Verification items for the finished model (mm, model axes). Face numbers are marked on the shaded views. A direction names the side the tool comes from. Coordinates: 2 decimals unless noted, no trailing zeros. Write each loop counter-clockwise with the first axis right and the second up, starting at its lowest first coordinate (ties: lowest second). Pieces come first, ordered by that corner, then holes. Notation, with made-up numbers: (8.25, 35) -> (17.25, 35) arc R18 cw to (17.25, 49) -> close; hole circle Ø1 at (9, 22.5). An arc over 180 degrees is marked (long way). Answer in a Markdown table with one row per item.
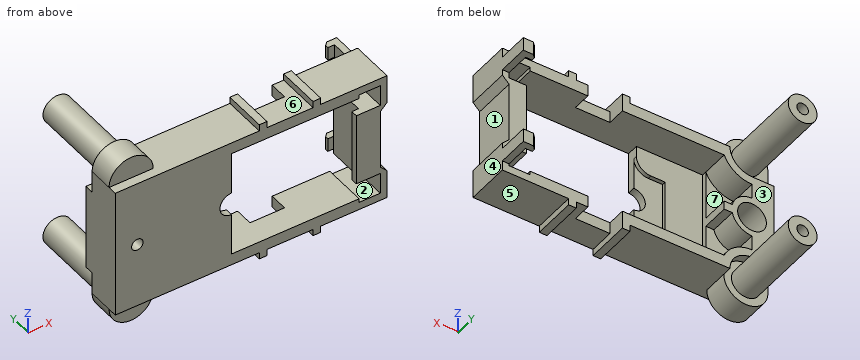
```python
from build123d import *

# Parameters (mm, degrees)
SKETCH1_W           = 35.941
SKETCH1_H           = 17.272
BOSS_EXTRUDE1_DEPTH = 5.715
SKETCH2_W           = 4.572
SKETCH2_H           = 2.413
CUT_EXTRUDE1_DEPTH  = 26.571900188
SKETCH3_W           = 4.699
SKETCH3_H           = 7.112
CUT_EXTRUDE2_DEPTH  = 21.740795338
SKETCH4_W           = 8.763
SKETCH4_H           = 14.224
CUT_EXTRUDE3_DEPTH  = 2.54
SKETCH4_2_W         = 8.763
SKETCH4_2_H         = 14.224
CUT_EXTRUDE4_DEPTH  = 4.191
SKETCH6_W           = 9.652
SKETCH6_H           = 0.8763
BOSS_EXTRUDE2_DEPTH = 0.8763
SKETCH7_W           = 0.889
SKETCH7_H           = 1.778
BOSS_EXTRUDE3_DEPTH = 4.064
SKETCH9_W           = 1.778
SKETCH9_H           = 0.8763
BOSS_EXTRUDE5_DEPTH = 0.8763
CHAMFER1_SIZE       = 0.43815
SKETCH11_W          = 1.016
SKETCH11_H          = 5.715
BOSS_EXTRUDE6_DEPTH = 0.8763
CUT_EXTRUDE5_DEPTH  = 0.508
CUT_EXTRUDE6_DEPTH  = 23.140751806
SKETCH20_W          = 5.842
SKETCH20_H          = 3.302
BOSS_EXTRUDE8_DEPTH = 4.318
CUT_EXTRUDE12_DEPTH = 1.2065
CUT_EXTRUDE13_DEPTH = 23.771103542
SKETCH26_R          = 1.905
SKETCH26_R_2        = 0.762
BOSS_EXTRUDE9_DEPTH = 11.049
SKETCH27_R          = 1.905
CUT_EXTRUDE14_DEPTH = 3.5687
SKETCH29_R          = 0.762
CUT_EXTRUDE15_DEPTH = 26.226244364


with BuildPart() as part:
    # Sketch1 → Boss-Extrude1 (new body)
    with BuildSketch(Plane(origin=(0, 0, 0), x_dir=(1, 0, 0), z_dir=(0, 1, 0))):
        Rectangle(SKETCH1_W, SKETCH1_H)
    extrude(amount=BOSS_EXTRUDE1_DEPTH)

    # Sketch2 → Cut-Extrude1 (cut, through all)
    with BuildSketch(Plane.XY.offset(8.636)):
        with Locations((4.3815, 4.5085)):
            Rectangle(SKETCH2_W, SKETCH2_H)
    extrude(amount=-CUT_EXTRUDE1_DEPTH, mode=Mode.SUBTRACT)

    # Sketch3 → Cut-Extrude2 (cut, through all)
    with BuildSketch(Plane(origin=(0, 5.715, 0), x_dir=(1, 0, 0), z_dir=(0, 1, 0))):
        with Locations((-0.254, 3.556)):
            Rectangle(SKETCH3_W, SKETCH3_H)
        Polygon((17.0815, 4.826), (17.0815, 7.62), (14.2875, 7.62), (14.2875, 7.112), (2.0955, 7.112), (2.0955, 0), (14.7955, 0), (14.7955, 4.826), align=None)
        Polygon((14.7955, -4.826), (14.7955, 0), (2.0955, 0), (2.0955, -7.112), (14.2875, -7.112), (14.2875, -7.62), (17.0815, -7.62), (17.0815, -4.826), align=None)
        with Locations((-0.254, -3.556)):
            Rectangle(SKETCH3_W, SKETCH3_H)
        Polygon((17.9705, 0), (17.0815, 0), (17.0815, -3.937), (17.9705, -4.826), align=None)
        Polygon((17.0815, 3.937), (17.0815, 0), (17.9705, 0), (17.9705, 4.826), align=None)
    extrude(amount=-CUT_EXTRUDE2_DEPTH, mode=Mode.SUBTRACT)

    # Sketch4 → Cut-Extrude3 (cut)
    with BuildSketch(Plane(origin=(0, 5.715, 0), x_dir=(1, 0, 0), z_dir=(0, 1, 0))):
        with Locations((-6.985, 0)):
            Rectangle(SKETCH4_W, SKETCH4_H)
    extrude(amount=-CUT_EXTRUDE3_DEPTH, mode=Mode.SUBTRACT)

    # Sketch4_2 → Cut-Extrude4 (cut)
    with BuildSketch(Plane(origin=(0, 5.715, 0), x_dir=(1, 0, 0), z_dir=(0, 1, 0))):
        with Locations((-6.985, 0)):
            Rectangle(SKETCH4_2_W, SKETCH4_2_H)
    extrude(amount=-CUT_EXTRUDE4_DEPTH, mode=Mode.SUBTRACT)

    # Sketch6 → Boss-Extrude2 (add)
    with BuildSketch(Plane.ZY.offset(-14.7955)):
        with Locations((0, 0.43815)):
            Rectangle(SKETCH6_W, SKETCH6_H)
    extrude(amount=BOSS_EXTRUDE2_DEPTH)

    # Sketch7 → Boss-Extrude3 (add)
    with BuildSketch(Plane(origin=(0, 5.715, 0), x_dir=(1, 0, 0), z_dir=(0, 1, 0))):
        with Locations((17.526, 6.470028065)):
            Rectangle(SKETCH7_W, SKETCH7_H)
        with Locations((17.526, -6.470028065)):
            Rectangle(SKETCH7_W, SKETCH7_H)
    extrude(amount=BOSS_EXTRUDE3_DEPTH)

    # Sketch9 → Boss-Extrude5 (add)
    with BuildSketch(Plane.ZY.offset(-17.0815)):
        with Locations((-6.470028065, 9.34085)):
            Rectangle(SKETCH9_W, SKETCH9_H)
        with Locations((6.470028065, 9.34085)):
            Rectangle(SKETCH9_W, SKETCH9_H)
    extrude(amount=BOSS_EXTRUDE5_DEPTH)

    # Chamfer1
    chamfer1_edges = [part.edges().sort_by_distance(p)[0] for p in [
        (16.2052, 9.779, -6.470028065),
        (16.2052, 9.779, 6.470028065),
    ]]
    chamfer(chamfer1_edges, length=CHAMFER1_SIZE)

    # Sketch11 → Boss-Extrude6 (add)
    with BuildSketch(Plane(origin=(0, 0, -8.636), x_dir=(-1, 0, 0), z_dir=(0, 0, -1))):
        with Locations((-1.5875, 2.8575)):
            Rectangle(SKETCH11_W, SKETCH11_H)
        with Locations((-8.6995, 2.8575)):
            Rectangle(SKETCH11_W, SKETCH11_H)
    boss_extrude6 = extrude(amount=BOSS_EXTRUDE6_DEPTH)

    # Mirror1: Boss-Extrude6 across plane
    add(boss_extrude6.mirror(Plane.XY))

    # Sketch12 → Cut-Extrude5 (cut)
    with BuildSketch(Plane(origin=(0, 1.524, 0), x_dir=(1, 0, 0), z_dir=(0, 1, 0))):
        with BuildLine():
            Line((-2.6035, -5.715), (-2.6035, 0))
            Line((-2.6035, 0), (-6.4135, 0))
            Line((-6.4135, 0), (-6.4135, -3.81))
            Line((-6.4135, -3.81), (-4.5085, -3.81))
            ThreePointArc((-4.5085, -3.81), (-3.161461582, -4.367961582), (-2.6035, -5.715))
        make_face()
        with BuildLine():
            Line((-6.4135, 0), (-2.6035, 0))
            Line((-2.6035, 0), (-2.6035, 5.715))
            ThreePointArc((-2.6035, 5.715), (-3.161461582, 4.367961582), (-4.5085, 3.81))
            Line((-4.5085, 3.81), (-6.4135, 3.81))
            Line((-6.4135, 3.81), (-6.4135, 0))
        make_face()
    extrude(amount=-CUT_EXTRUDE5_DEPTH, mode=Mode.SUBTRACT)

    # Sketch13 → Cut-Extrude6 (cut, through all)
    with BuildSketch(Plane(origin=(0, 1.016, 0), x_dir=(1, 0, 0), z_dir=(0, 1, 0))):
        with BuildLine():
            Line((-2.6035, -1.524), (-2.6035, 1.524))
            ThreePointArc((-2.6035, 1.524), (-4.1275, 0), (-2.6035, -1.524))
        make_face()
    extrude(amount=-CUT_EXTRUDE6_DEPTH, mode=Mode.SUBTRACT)

    # Sketch20 → Boss-Extrude8 (add)
    with BuildSketch(Plane.XY.offset(8.636)):
        with Locations((-15.0495, 2.8575)):
            Rectangle(SKETCH20_W, SKETCH20_H)
    boss_extrude8 = extrude(amount=BOSS_EXTRUDE8_DEPTH)

    # Mirror5: Boss-Extrude8 across plane
    add(boss_extrude8.mirror(Plane.XY))

    # Sketch23 → Cut-Extrude12 (cut)
    with BuildSketch(Plane(origin=(0, 5.715, 0), x_dir=(1, 0, 0), z_dir=(0, 1, 0))):
        with BuildLine():
            Line((-15.0495, -5.715), (-17.9705, -5.715))
            Line((-17.9705, -5.715), (-17.9705, -8.636))
            Line((-17.9705, -8.636), (-12.1285, -8.636))
            ThreePointArc((-12.1285, -8.636), (-12.984041092, -6.570541092), (-15.0495, -5.715))
        make_face()
    cut_extrude12 = extrude(amount=-CUT_EXTRUDE12_DEPTH, mode=Mode.SUBTRACT)

    # Mirror8: Cut-Extrude12 across plane
    add(cut_extrude12.mirror(Plane.XY), mode=Mode.SUBTRACT)

    # Sketch25 → Cut-Extrude13 (cut, through all)
    with BuildSketch(Plane(origin=(0, 4.5085, 0), x_dir=(1, 0, 0), z_dir=(0, 1, 0))):
        with BuildLine():
            Line((-12.1285, -8.636), (-12.1285, -12.954))
            Line((-12.1285, -12.954), (-17.9705, -12.954))
            Line((-17.9705, -12.954), (-17.9705, -8.636))
            ThreePointArc((-17.9705, -8.636), (-15.0495, -11.557), (-12.1285, -8.636))
        make_face()
    cut_extrude13 = extrude(amount=-CUT_EXTRUDE13_DEPTH, mode=Mode.SUBTRACT)

    # Mirror9: Cut-Extrude13 across plane
    add(cut_extrude13.mirror(Plane.XY), mode=Mode.SUBTRACT)

    # Sketch26 → Boss-Extrude9 (add)
    with BuildSketch(Plane(origin=(0, 4.5085, 0), x_dir=(1, 0, 0), z_dir=(0, 1, 0))):
        with Locations((-15.0495, -8.636)):
            Circle(SKETCH26_R)
        with Locations(Location((-15.0495, -8.636, 0), (0, 0, 180))):
            Circle(SKETCH26_R_2, mode=Mode.SUBTRACT)
    boss_extrude9 = extrude(amount=BOSS_EXTRUDE9_DEPTH)

    # Mirror10: Boss-Extrude9 across plane
    add(boss_extrude9.mirror(Plane.XY))

    # Sketch27 → Cut-Extrude14 (cut)
    with BuildSketch(Plane(origin=(0, 5.715, 0), x_dir=(1, 0, 0), z_dir=(0, 1, 0))):
        with BuildLine():
            Line((-12.44445168, 0.5715), (-11.3665, 0.5715))
            Line((-11.3665, 0.5715), (-11.3665, 7.112))
            ThreePointArc((-11.3665, 7.112), (-12.834481127, 5.322277563), (-15.0495, 4.650141874))
            Line((-15.0495, 4.650141874), (-15.0495, 2.667))
            ThreePointArc((-15.0495, 2.667), (-13.377869284, 2.078109658), (-12.44445168, 0.5715))
        make_face()
        with BuildLine():
            Line((-11.3665, -7.112), (-11.3665, -0.5715))
            Line((-11.3665, -0.5715), (-12.44445168, -0.5715))
            ThreePointArc((-12.44445168, -0.5715), (-13.377869284, -2.078109658), (-15.0495, -2.667))
            Line((-15.0495, -2.667), (-15.0495, -4.650141874))
            ThreePointArc((-15.0495, -4.650141874), (-12.834481127, -5.322277563), (-11.3665, -7.112))
        make_face()
        with Locations(Location((-15.0495, 0, 0), (0, 0, 270))):
            Circle(SKETCH27_R)
    extrude(amount=-CUT_EXTRUDE14_DEPTH, mode=Mode.SUBTRACT)

    # Sketch29 → Cut-Extrude15 (cut, through all)
    with BuildSketch(Plane(origin=(0, 2.1463, 0), x_dir=(1, 0, 0), z_dir=(0, 1, 0))):
        with Locations(Location((-15.0495, 0, 0), (0, 0, 270))):
            Circle(SKETCH29_R)
    extrude(amount=-CUT_EXTRUDE15_DEPTH, mode=Mode.SUBTRACT)


solid = part.part
```
1. Sectioned sample at B-B, the plane z = 3.25. Record the cut outline in (x, y) (1 decimal), and give its area (4 significant figures).
Findings below:
| item | result |
|---|---|
| outline | (-18, 0) -> (-2.6, 0) -> (-2.6, 1) -> (-6.4, 1) -> (-6.4, 1.5) -> (-11.4, 1.5) -> (-11.4, 2.1) -> (-15, 2.1) -> (-15, 5.7) -> (-18, 5.7) -> close; (13.9, 0) -> (17.1, 0) -> (17.1, 5.7) -> (14.8, 5.7) -> (14.8, 0.9) -> (13.9, 0.9) -> close |
| area | 49.85 mm² |
2. Access from +Z, -Z, +X, -X, +Y, -Y to the whole of each face (thin tool, end or side, straight path). Record for the marked faces 1, 2, 3 and 4.
Findings below:
| item | result |
|---|---|
| face 1 | +X, +Y, -Y |
| face 2 | +Y, -Y |
| face 3 | +Y |
| face 4 | +Z, -Z, +X, +Y, -Y |
3. Sectioned sample at C-C, the plane x = 3. Record the cut outline in (y, z), and give its area (3 significant figures).
Findings below:
| item | result |
|---|---|
| outline | (0, -8.64) -> (3.3, -8.64) -> (3.3, -7.11) -> (0, -7.11) -> close; (0, 7.11) -> (3.3, 7.11) -> (3.3, 8.64) -> (0, 8.64) -> close |
| area | 10.1 mm² |
4. Release check for a two-part mould opening along Z. For the marked faces 5, 6 and 7 record: released by +Z, released by -Z, zero draft, split by the parting line, or undercut.
Findings below:
| item | result |
|---|---|
| face 5 | released by -Z |
| face 6 | released by +Z |
| face 7 | undercut |
5. Sectioned sample at A-A, the plane y = 6.5. Record the cut outline in (x, z) (1 decimal), and give its area (3 significant figures).
Findings below:
| item | result |
|---|---|
| outline | circle Ø3.8 at (-15, -8.6); circle Ø3.8 at (-15, 8.6); (17.1, -7.4) -> (18, -7.4) -> (18, -5.6) -> (17.1, -5.6) -> close; (17.1, 5.6) -> (18, 5.6) -> (18, 7.4) -> (17.1, 7.4) -> close; hole circle Ø1.5 at (-15, -8.6); hole circle Ø1.5 at (-15, 8.6) |
| area | 22.3 mm² |
6. Material ranges on probe 1 along X at (y, z) = (3.85, 0); probe 2 along Z at (x, y) = (-15, 3.5); probe 3 along X at (y, z) = (1.7, 0), recorded low to high. Write a range as from..to.
Findings below:
| item | result |
|---|---|
| probe 1 | x = -17.97..-16.95, -13.14..-11.37, 14.8..17.08 |
| probe 2 | z = -11.56..-4.65, -2.67..-1.9, 1.9..2.67, 4.65..11.56 |
| probe 3 | x = -17.97..-15.81, -14.29..-11.37, 14.8..17.08 |
7. Sectioned sample at D-D, the plane z = 0. Record the cut outline in (x, y) (1 decimal).
Findings below:
| item | result |
|---|---|
| outline | (-18, 0) -> (-15.8, 0) -> (-15.8, 2.1) -> (-17, 2.1) -> (-17, 5.7) -> (-18, 5.7) -> close; (-14.3, 0) -> (-4.1, 0) -> (-4.1, 1) -> (-6.4, 1) -> (-6.4, 1.5) -> (-11.4, 1.5) -> (-11.4, 5.7) -> (-13.1, 5.7) -> (-13.1, 2.1) -> (-14.3, 2.1) -> close; (13.9, 0) -> (17.1, 0) -> (17.1, 5.7) -> (14.8, 5.7) -> (14.8, 0.9) -> (13.9, 0.9) -> close |
8. Go/stop test with flat-tipped pins: pin 1 (4 mm diameter, centred on y = 13.5, z = -5, fed in from +X); pin 2 (2 mm diameter, centred on x = 1.5, y = 2.5, fed in from +Z); pin 3 (4.5 mm diameter, centred on x = 5, y = 3, fed in from +Z). Record where each tip stops, or that it passes through.
Findings below:
| item | result |
|---|---|
| pin 1 | stops at x = -14.07 |
| pin 2 | stops at z = 9.51 |
| pin 3 | stops at z = 8.64 |
